Geometry: final body of the model. Coordinates: model frame, mm. Give positions to 0.01 mm unless a question says otherwise; leave off trailing zeros. Order: outer loops, then holes, each group sorted by start corner. A loop starts at its lowest first (then second) coordinate and runs counter-clockwise, first axis right, second up. Notation, with made-up numbers: (11, 87) -> (30, 87) arc R29 cw to (30, 109) -> close; hole circle Ø6 at (17.25, -13.5). An arc over 180 degrees is marked (long way). One line per question, with ' | ' between items.
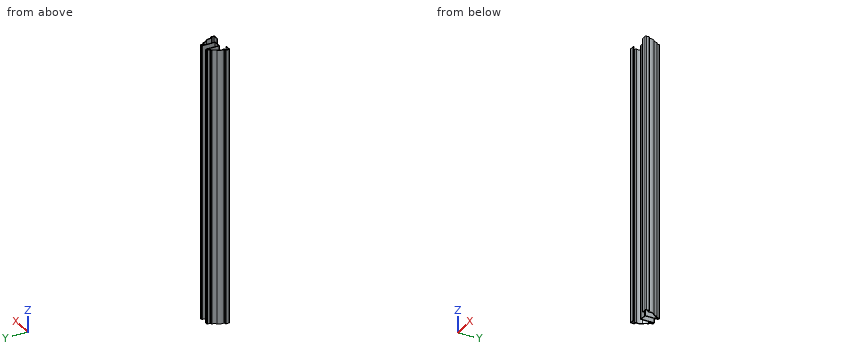
from build123d import *

# Parameters (mm, degrees)
EXTRUDE_THIN1_DEPTH = 396.875
FILLET1_R           = 1.016


with BuildPart() as part:
    # Sketch1 → Extrude-Thin1 (new body)
    with BuildSketch(Plane.XY):
        with BuildLine():
            Line((-11.90625, 0), (-19.84375, 0))
            Line((-19.84375, 0), (-19.84375, 6.35))
            Line((-19.84375, 6.35), (-16.611859403, 6.35))
            ThreePointArc((-16.611859403, 6.35), (-16.819864191, 11.185113028), (-14.420873366, 15.388257922))
            ThreePointArc((-14.420873366, 15.388257922), (-12.164462393, 18.51520612), (-11.1125, 22.225))
            Line((-11.1125, 22.225), (-8.73125, 22.225))
            Line((-8.73125, 22.225), (-8.73125, 26.9875))
            Line((-8.73125, 26.9875), (-4.7625, 26.9875))
            Line((-4.7625, 26.9875), (-4.7625, 7.9375))
            Line((-4.7625, 7.9375), (4.7625, 7.9375))
            Line((4.7625, 7.9375), (4.7625, 26.9875))
            Line((4.7625, 26.9875), (8.73125, 26.9875))
            Line((8.73125, 26.9875), (8.73125, 22.225))
            Line((8.73125, 22.225), (11.1125, 22.225))
            ThreePointArc((11.1125, 22.225), (12.164462393, 18.51520612), (14.420873366, 15.388257922))
            ThreePointArc((14.420873366, 15.388257922), (16.819864191, 11.185113028), (16.611859403, 6.35))
            Line((16.611859403, 6.35), (19.84375, 6.35))
            Line((19.84375, 6.35), (19.84375, 0))
            Line((19.84375, 0), (11.90625, 0))
            Line((11.90625, 0), (11.90625, 1.016))
            Line((11.90625, 1.016), (18.82775, 1.016))
            Line((18.82775, 1.016), (18.82775, 5.334))
            Line((18.82775, 5.334), (15.052239099, 5.334))
            ThreePointArc((15.052239099, 5.334), (15.971237356, 10.225128152), (13.712626283, 14.659806091))
            ThreePointArc((13.712626283, 14.659806091), (11.458524166, 17.661660911), (10.230316486, 21.209))
            Line((10.230316486, 21.209), (7.71525, 21.209))
            Line((7.71525, 21.209), (7.71525, 25.9715))
            Line((7.71525, 25.9715), (5.7785, 25.9715))
            Line((5.7785, 25.9715), (5.7785, 6.9215))
            Line((5.7785, 6.9215), (-5.7785, 6.9215))
            Line((-5.7785, 6.9215), (-5.7785, 25.9715))
            Line((-5.7785, 25.9715), (-7.71525, 25.9715))
            Line((-7.71525, 25.9715), (-7.71525, 21.209))
            Line((-7.71525, 21.209), (-10.230316486, 21.209))
            ThreePointArc((-10.230316486, 21.209), (-11.458524166, 17.661660911), (-13.712626283, 14.659806091))
            ThreePointArc((-13.712626283, 14.659806091), (-15.971237356, 10.225128152), (-15.052239099, 5.334))
            Line((-15.052239099, 5.334), (-18.82775, 5.334))
            Line((-18.82775, 5.334), (-18.82775, 1.016))
            Line((-18.82775, 1.016), (-11.90625, 1.016))
            Line((-11.90625, 1.016), (-11.90625, 0))
        make_face()
    extrude(amount=-EXTRUDE_THIN1_DEPTH)

    # Fillet1
    fillet1_edges = [part.edges().sort_by_distance(p)[0] for p in [
        (-19.84375, 0, -198.4375),
        (-19.84375, 6.35, -198.4375),
        (-11.1125, 22.225, -198.4375),
        (-8.73125, 26.9875, -198.4375),
        (-4.7625, 26.9875, -198.4375),
        (4.7625, 26.9875, -198.4375),
        (8.73125, 26.9875, -198.4375),
        (11.1125, 22.225, -198.4375),
        (19.84375, 6.35, -198.4375),
        (19.84375, 0, -198.4375),
        (15.052239099, 5.334, -198.4375),
        (7.71525, 21.209, -198.4375),
        (5.7785, 6.9215, -198.4375),
        (-5.7785, 6.9215, -198.4375),
        (-7.71525, 21.209, -198.4375),
        (-15.052239099, 5.334, -198.4375),
    ]]
    fillet(fillet1_edges, radius=FILLET1_R)


solid = part.part
1) Material intervals for probe 1 along X at (y, z) = (9.5, -360); probe 2 along X at (y, z) = (10, -39); probe 3 along X at (y, z) = (2.5, -182.5), sorted ascending. Write a range as from..to.
Check result:
probe 1: x = -17.06..-16.04, -5.78..-4.76, 4.76..5.78, 16.04..17.06 | probe 2: x = -17.02..-16, -5.78..-4.76, 4.76..5.78, 16..17.02 | probe 3: x = -19.84..-18.83, 18.83..19.84
2) Section A-A on y = 11.25. Return loops of the section in (x, z) (1 decimal).
Check result:
outline: (-16.8, -396.9) -> (-15.8, -396.9) -> (-15.8, 0) -> (-16.8, 0) -> close; (-5.8, -396.9) -> (-4.8, -396.9) -> (-4.8, 0) -> (-5.8, 0) -> close; (4.8, -396.9) -> (5.8, -396.9) -> (5.8, 0) -> (4.8, 0) -> close; (15.8, -396.9) -> (16.8, -396.9) -> (16.8, 0) -> (15.8, 0) -> close
3) Contact query for flat-ended pins moving along their axis: pin 1 Ø4 at (y, z) = (24.5, -207.5) entering from -X; pin 2 Ø0.7 at (x, z) = (9.5, -221) entering from -Y; pin 3 Ø3.5 at (x, z) = (-16, -179) entering from +Y. Output: stop coordinate, or through.
Check result:
pin 1: stops at x = -8.73 | pin 2: stops at y = 21.21 | pin 3: stops at y = 15.56
4) Section B-B on x = 1. Return loops of the section in (y, z) (1 decimal).
Check result:
outline: (6.9, -396.9) -> (7.9, -396.9) -> (7.9, 0) -> (6.9, 0) -> close
